Geometry: see drawing. Coordinates: mm, zero at the bounding-box minimum. A direction names the side the tool comes from. Round coordinates to 2 decimals unless told otherwise and drop trailing zeros. Write each loop counter-clockwise with the first axis right and the second up, starting at its lowest first coordinate (ties: lowest second). Pieces come first, ordered by that corner, then holes. Notation, with made-up numbers: (-36.5, -26.75) -> (-14.5, -26.75) arc R32 cw to (-14.5, 3.25) -> close; hole circle Ø6 at (-4.75, 66). An arc over 180 degrees is marked (long way). Write item = value, one per line.
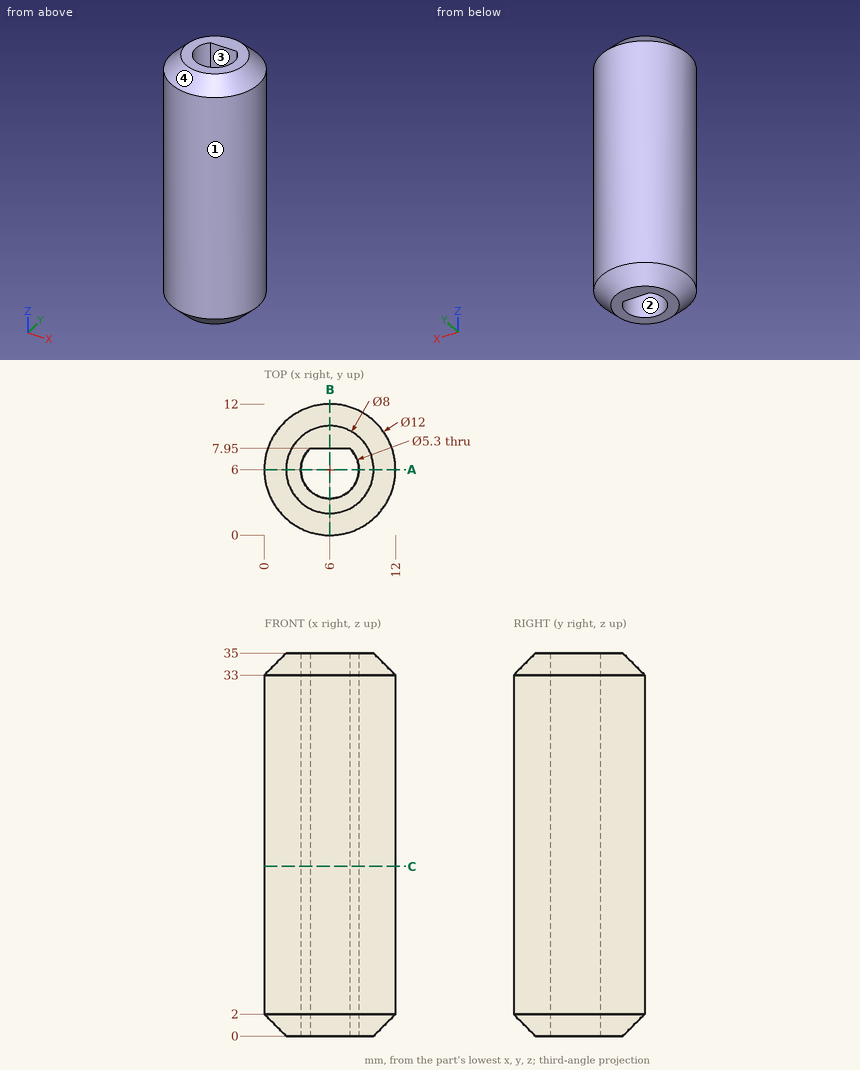
1) Cut plane C-C (z = 15.5). Return the cut outline in (x, y), and give its area (3 significant figures).
Solutions:
outline = circle Ø12 at (6, 6); hole (4.21, 7.95) arc R2.65 ccw (long way) to (7.79, 7.95) -> close
area = 92.8 mm^2
2) Cut plane A-A (y = 6). Return the cut outline in (x, z), and give its area (4 significant figures).
Solutions:
outline = (0, 2) -> (2, 0) -> (3.35, 0) -> (3.35, 35) -> (2, 35) -> (0, 33) -> close; (8.65, 0) -> (10, 0) -> (12, 2) -> (12, 33) -> (10, 35) -> (8.65, 35) -> close
area = 226.5 mm^2
3) Cut plane B-B (x = 6). Return the cut outline in (y, z).
Solutions:
outline = (0, 2) -> (2, 0) -> (3.35, 0) -> (3.35, 35) -> (2, 35) -> (0, 33) -> close; (7.95, 0) -> (10, 0) -> (12, 2) -> (12, 33) -> (10, 35) -> (7.95, 35) -> close
4) Access query for the marked faces 3 and 4. Directions: +Z, -Z, +X, -X, +Y, -Y. A direction counts if a zero-diameter tool reaches every point of the face in a straight line with its end or side. Return the directions, or none.
Solutions:
face_3 = +Z, -Z
face_4 = +Z
5) First-contact query: P1, Ø5, axis at x = 1.5, z = 9, coming from the -Y side; P2, Ø3, axis at x = 2.5, z = 11, coming from the +Y side; P3, Ø2, axis at x = 1.5, z = 31.5, coming from the -Y side. Flat tips, straight axial feed; report the tip coordinate or a pass-through.
Solutions:
P1 = 0.34
P2 = 11.66
P3 = 1.13
6) Line query: L1, parallel to Y at x = 6, z = 28.5; L2, parallel to Y at x = 6, z = 33.5; L3, parallel to X at y = 6.5, z = 28.5. Output: solid intervals per line, ascending. Write a range as from..to.
Solutions:
L1 = 0..3.35, 7.95..12
L2 = 0.5..3.35, 7.95..11.5
L3 = 0.02..3.4, 8.6..11.98
7) Draft query along Y for the marked faces 1 and 2. Return one class per face: +Y half, -Y half, draft (parallel to the pull), parting line (faces both ways), or undercut.
Solutions:
face_1 = parting line
face_2 = undercut
